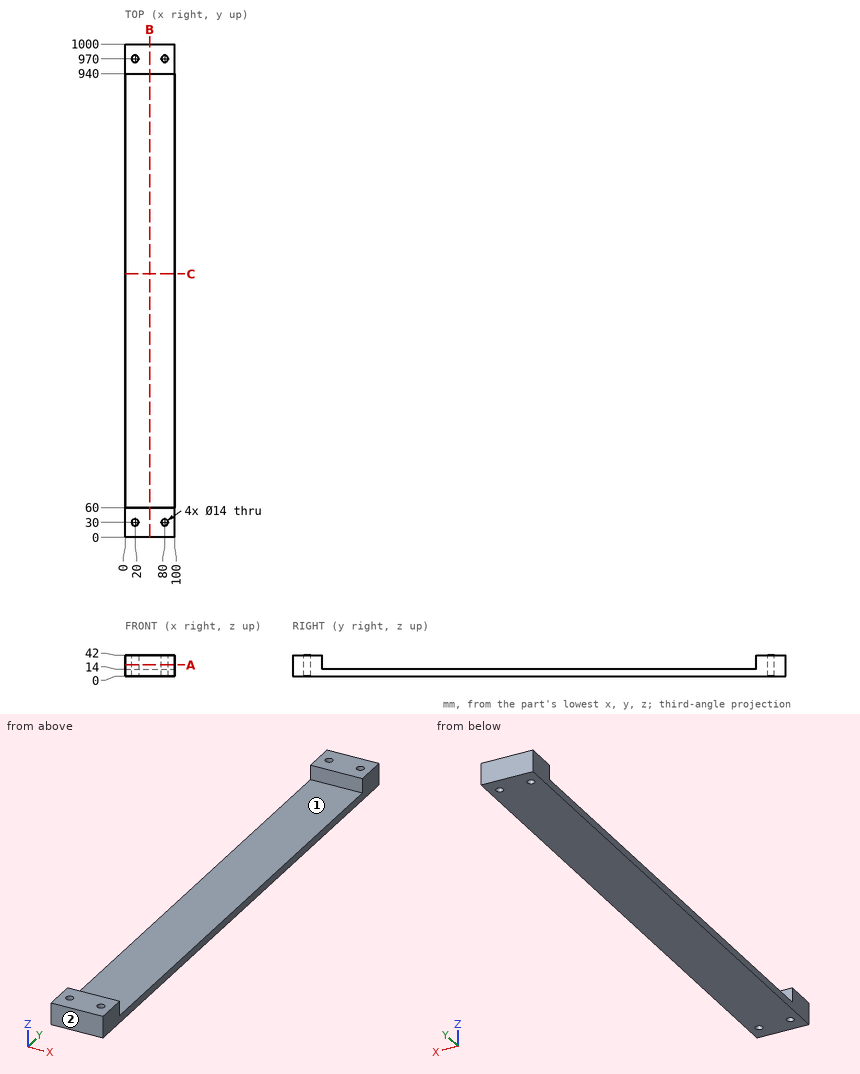
Answer from the drawing. Dimensions are ordinates in mm from the lowest x, y and z of the part. A direction names the side the tool comes from. Give positions to 0.01 mm unless a question says otherwise; leave off trailing zeros. Write each loop counter-clockwise with the first axis right and the second up, starting at its lowest first coordinate (ties: lowest second). Pieces come first, ordered by that corner, then holes. Notation, with made-up numbers: (41, 63.5) -> (57, 63.5) arc R21 cw to (57, 101.5) -> close; hole circle Ø5 at (85, 48.5). An arc over 180 degrees is marked (long way). Use a Markdown table: item, result.
(1) Section C-C, the plane y = 534 is taken. Determine the outline of the cut face in (x, z).
Return value:
| item | result |
|---|---|
| outline | (0, 0) -> (100, 0) -> (100, 14) -> (0, 14) -> close |
(2) For the marked faces 1 and 2, determine the directions among +Z, -Z, +X, -X, +Y, -Y from which every point of the face is accessible in a straight line to the end or side of a thin tool.
Return value:
| item | result |
|---|---|
| face 1 | +Z, +X, -X |
| face 2 | +Z, -Z, +X, -X, -Y |
(3) A flat-ended cylindrical pin translates along its axis: P1, Ø8.5, axis at x = 80, y = 970, coming from the +Z side. Find the tip coordinate at first contact, or state that the pin passes through.
Return value:
| item | result |
|---|---|
| P1 | through |
(4) Section B-B, the plane x = 49.5 is taken. Determine the outline of the cut face in (y, z).
Return value:
| item | result |
|---|---|
| outline | (0, 0) -> (1000, 0) -> (1000, 42) -> (940, 42) -> (940, 14) -> (60, 14) -> (60, 42) -> (0, 42) -> close |
(5) Find the intervals of material crossed by probe 1 along X at (y, z) = (970, 32); probe 2 along Y at (x, z) = (20, 18); probe 3 along Y at (x, z) = (25.5, 11.5), in increasing order. Write a range as from..to.
Return value:
| item | result |
|---|---|
| probe 1 | 0..13, 27..73, 87..100 |
| probe 2 | 0..23, 37..60, 940..963, 977..1000 |
| probe 3 | 0..25.67, 34.33..965.67, 974.33..1000 |
(6) Section A-A, the plane z = 22.5 is taken. Determine the outline of the cut face in (x, y).
Return value:
| item | result |
|---|---|
| outline | (0, 0) -> (100, 0) -> (100, 60) -> (0, 60) -> close; (0, 940) -> (100, 940) -> (100, 1000) -> (0, 1000) -> close; hole circle Ø14 at (20, 30); hole circle Ø14 at (20, 970); hole circle Ø14 at (80, 30); hole circle Ø14 at (80, 970) |
